from build123d import *

# Parameters (mm, degrees)
F1_DEPTH = 10
F2_R     = 1.75
F3_DEPTH = 4
F5_DEPTH = 2.1
F6_R     = 4.8
F7_SIZE  = 1
F8_SIZE  = 0.5


with BuildPart() as f1:
    # F0 (on Right) → F1 (new body)
    with BuildSketch(Plane.YZ):
        Polygon((-11.8, 4), (-11.8, 0), (0, 0), (0, 10), (-4, 4), align=None)
    extrude(amount=F1_DEPTH)

    # F2 (on face) → F3 (cut, through all)
    with BuildSketch(Plane(origin=(0, 0, 0), x_dir=(1, 0, 0), z_dir=(0, 0, -1))):
        with Locations((5, 7.8)):
            Circle(F2_R)
    extrude(amount=-F3_DEPTH, mode=Mode.SUBTRACT)

    # F4 (on face) → F5 (join)
    with BuildSketch(Plane(origin=(0, 0, 0), x_dir=(-1, 0, 0), z_dir=(0, 1, 0))):
        Polygon((-7, 6), (-9, 0), (-1, 0), (-3, 6), align=None)
    extrude(amount=F5_DEPTH)

    # F6
    f6_edges = [f1.edges().sort_by_distance(p)[0] for p in [
        (0, -11.8, 2),
        (10, -11.8, 2),
    ]]
    fillet(f6_edges, radius=F6_R)

    # F7
    f7_edges = [f1.edges().sort_by_distance(p)[0] for p in [
        (0, -5.5, 4),
        (0, -2, 7),
        (10, -2, 7),
    ]]
    chamfer(f7_edges, length=F7_SIZE)

    # F8
    f8_edges = [f1.edges().sort_by_distance(p)[0] for p in [
        (2, 2.1, 3),
        (5, 2.1, 6),
        (8, 2.1, 3),
    ]]
    chamfer(f8_edges, length=F8_SIZE)


solid = f1.part
The model under review builds one solid part; all positions refer to its coordinate system, in mm. A direction names the side the tool comes from. Round coordinates to 2 decimals unless told otherwise and drop trailing zeros. Write each loop counter-clockwise with the first axis right and the second up, starting at its lowest first coordinate (ties: lowest second). Pieces come first, ordered by that corner, then holes. Notation, with made-up numbers: (3.5, 1) -> (20.5, 1) arc R28 ccw to (20.5, 22) -> close; hole circle Ø7 at (15.25, 58). An arc over 180 degrees is marked (long way). Answer as a JSON object with one key per item and string values.
1. We need section B-B on z = 2. State the section outline as (x, y) points.
Results found:
{"outline": "(0, -7) arc R4.8 ccw to (4.8, -11.8) -> (5.2, -11.8) arc R4.8 ccw to (10, -7) -> (10, 0) -> (8.33, 0) -> (8.33, 1.6) -> (7.81, 2.1) -> (2.19, 2.1) -> (1.67, 1.6) -> (1.67, 0) -> (0, 0) -> close; hole circle Ø3.5 at (5, -7.8)"}
2. We need section D-D on z = 5.75. State the section outline as (x, y) points.
Results found:
{"outline": "(0, -1.63) -> (1, -2.83) -> (9, -2.83) -> (10, -1.63) -> (10, 0) -> (7.08, 0) -> (7.08, 1.6) -> (6.82, 1.85) -> (3.18, 1.85) -> (2.92, 1.6) -> (2.92, 0) -> (0, 0) -> close"}
3. We need section A-A on x = 5. State the section outline as (y, z) points, and give its area (3 significant figures).
Results found:
{"outline": "(-11.8, 0) -> (-9.55, 0) -> (-9.55, 4) -> (-10.8, 4) -> (-11.8, 3) -> close; (-6.05, 0) -> (2.1, 0) -> (2.1, 5.5) -> (1.6, 6) -> (0, 6) -> (0, 10) -> (-4, 4) -> (-6.05, 4) -> close", "area": "57.2 mm^2"}
4. The part is to be moulded in two halves that separate along Y. For faces 1 (the face through (10, -3, 2)), 2 (the face through (3.71, -8.98, 1.97)), 3 (the face through (5, 2.1, 2)), 4 (the face through (0.51, -1.71, 6.55)), say which applies: pulls with the +Y half, pulls with the -Y half, needs draft (parallel to the pull), parting line crosses it, or undercut.
Results found:
{"face 1": "needs draft", "face 2": "undercut", "face 3": "pulls with the +Y half", "face 4": "pulls with the -Y half"}
5. We need section C-C on y = -4.5. State the section outline as (x, z) points.
Results found:
{"outline": "(0, 0) -> (10, 0) -> (10, 3) -> (9, 4) -> (1, 4) -> (0, 3) -> close"}
6. To check wall thickness, follow line 1 along Y through (x, z) = (5, 2.3); line 2 along Z through (x, y) = (3.75, -4.75); line 3 along Z through (x, y) = (3.25, 0.25). State the ranges of each line that lie inside material, in increasing order.
Results found:
{"line 1": "y = -11.8 to -9.55, -6.05 to 2.1", "line 2": "z = 0 to 4", "line 3": "z = 0 to 6"}
7. Clearance check with flat-ended pins moving along their axes: pin 1 (0.8 mm diameter, centred on x = 5, y = 0.5, fed in from +Z); pin 2 (3 mm diameter, centred on x = 6.5, y = -9.5, fed in from +Z); pin 3 (3 mm diameter, centred on x = 5, y = -7.8, fed in from -Z); pin 4 (6 mm diameter, centred on x = 8, z = 8, fed in from -Y). State where each tip first meets the part, or that it passes through.
Results found:
{"pin 1": "stops at z = 6", "pin 2": "stops at z = 4", "pin 3": "passes through", "pin 4": "stops at y = -3.33"}
8. Machinability: for faces 5 (the face through (0.5, -5.2, 3.5)), 6 (the face through (5, 1, 6)), 7 (the face through (9.5, -5.3, 3.5)), 8 (the face through (4.9, -5.8, 4)), 9 (the face through (5, 0, 7)), which of the approach directions +Z, -Z, +X, -X, +Y, -Y give a long, thin tool a straight path to every point of the face, cutting with its end or side? Answer none if there is none.
Results found:
{"face 5": "+Z, -X, -Y", "face 6": "+Z, +X, -X, +Y", "face 7": "+Z, +X, -Y", "face 8": "+Z, +X, -X, -Y", "face 9": "+Z, +Y"}
